Check sheet for the modelled part. Datum: model origin and axes. Units: mm. A direction names the side the tool comes from. Coordinates: 2 decimals unless noted, no trailing zeros. Write each loop counter-clockwise with the first axis right and the second up, starting at its lowest first coordinate (ties: lowest second). Pieces come first, ordered by that corner, then holes. Notation, with made-up numbers: (51, 18) - (80, 18) arc R19 ccw to (80, 24) - close; hole circle Ø4 at (-24.5, 40). An arc over 180 degrees is marked (long way). Answer as CSV lines item,"result". Start each with the question number.
from build123d import *

# Parameters (mm, degrees)
SKETCH1_W               = 25
SKETCH1_H               = 10
BOSS_EXTRUDE1_DEPTH     = 3
SKETCH2_R               = 1.25
CUT_EXTRUDE1_DEPTH      = 10
SKETCH3_W               = 10
SKETCH3_H               = 3
BOSS_EXTRUDE2_DEPTH     = 3
SKETCH4_W               = 3
SKETCH4_H               = 19.36
BOSS_EXTRUDE3_DEPTH     = 10
BOSS_EXTRUDE4_DEPTH     = 3
SKETCH6_W               = 3
SKETCH6_H               = 25
BOSS_EXTRUDE5_DEPTH     = 23
SKETCH7_W               = 3
SKETCH7_H               = 15.439035089
BOSS_EXTRUDE6_DEPTH     = 5
BOSS_EXTRUDE7_DEPTH     = 2.9
BOSS_EXTRUDE8_DEPTH     = 10
CUT_EXTRUDE2_DEPTH      = 10
CUT_EXTRUDE3_DEPTH      = 42.797000958
CUT_EXTRUDE3_DEPTH_BACK = 42.797000958
SKETCH11_R              = 1.25
SKETCH12_R              = 1.6
CUT_EXTRUDE4_DEPTH      = 40


with BuildPart() as part:
    # Sketch1 → Boss-Extrude1 (new body)
    with BuildSketch(Plane(origin=(0, 0, 0), x_dir=(1, 0, 0), z_dir=(0, 1, 0))):
        Rectangle(SKETCH1_W, SKETCH1_H)
    extrude(amount=BOSS_EXTRUDE1_DEPTH)

    # Sketch2 → Cut-Extrude1 (cut)
    with BuildSketch(Plane(origin=(0, 3, 0), x_dir=(1, 0, 0), z_dir=(0, 1, 0))):
        with Locations(Location((-4.894136616, -1.366933975, 0), (0, 0, 270))):
            Circle(SKETCH2_R)
        with Locations(Location((4.605863384, -1.366933975, 0), (0, 0, 270))):
            Circle(SKETCH2_R)
    extrude(amount=-CUT_EXTRUDE1_DEPTH, mode=Mode.SUBTRACT)

    # Sketch3 → Boss-Extrude2 (add)
    with BuildSketch(Plane.ZY.offset(12.5)):
        with Locations((0, 1.5)):
            Rectangle(SKETCH3_W, SKETCH3_H)
    extrude(amount=BOSS_EXTRUDE2_DEPTH)

    # Sketch4 → Boss-Extrude3 (add)
    with BuildSketch(Plane(origin=(0, 0, -5), x_dir=(-1, 0, 0), z_dir=(0, 0, -1))):
        with Locations((14, -9.68)):
            Rectangle(SKETCH4_W, SKETCH4_H)
    extrude(amount=-BOSS_EXTRUDE3_DEPTH)

    # Sketch5 → Boss-Extrude4 (add)
    with BuildSketch(Plane.ZY.offset(15.5)):
        Polygon((5, -19.36), (5, -22.36), (-17.439050417, -22.36), (-20.439050417, -22.36), (-20.439050417, -19.359965116), (-17.439050417, -19.359965116), align=None)
    extrude(amount=-BOSS_EXTRUDE4_DEPTH)

    # Sketch6 → Boss-Extrude5 (add)
    with BuildSketch(Plane(origin=(-12.5, 0, 0), x_dir=(0, 0, -1), z_dir=(1, 0, 0))):
        with Locations((18.939050417, -19.359753222)):
            Rectangle(SKETCH6_W, SKETCH6_H)
    extrude(amount=BOSS_EXTRUDE5_DEPTH)


with BuildPart() as boss_extrude6_tool:
    # Sketch7 → Boss-Extrude6 (new body)
    with BuildSketch(Plane(origin=(0, -19.359992227, -3.0098e-05), x_dir=(1, 0, 0), z_dir=(0, 0.9999999999987916, 1.5546330463646684e-06))):
        with Locations((-14, 12.719522209)):
            Rectangle(SKETCH7_W, SKETCH7_H)
    extrude(amount=BOSS_EXTRUDE6_DEPTH)


with BuildPart() as part_1:
    add(part.part)


with BuildPart() as part_2:
    # Boss-Extrude6: joined with boss_extrude6_tool
    add(part_1.part.fuse(boss_extrude6_tool.part, tol=0.00001))

    # Sketch8 → Boss-Extrude7 (add)
    with BuildSketch(Plane(origin=(-12.5, 0, 0), x_dir=(0, 0, -1), z_dir=(1, 0, 0))):
        Polygon((17.439050417, -22.36), (-5, -22.36), (-5, 0), (5, 0), (5.000026988, -14.359984454), (17.439050417, -14.359962784), align=None)
    extrude(amount=BOSS_EXTRUDE7_DEPTH)

    # Sketch9 → Boss-Extrude8 (add)
    with BuildSketch(Plane(origin=(0, 0, -5), x_dir=(-1, 0, 0), z_dir=(0, 0, -1))):
        Polygon((1, 1.140246778), (15.5, 1.140246778), (15.5, 4.140246778), (-12.5, 4.140246778), (-12.5, 1.140246778), align=None)
    extrude(amount=-BOSS_EXTRUDE8_DEPTH)

    # Sketch10 → Cut-Extrude2 (cut)
    with BuildSketch(Plane(origin=(0, 0, -5), x_dir=(-1, 0, 0), z_dir=(0, 0, -1))):
        Polygon((-10.464750731, 1.14), (9.6, 1.14), (9.6, 0), (-12.5, 0), (-12.5, 1.14), align=None)
    extrude(amount=-CUT_EXTRUDE2_DEPTH, mode=Mode.SUBTRACT)

    # Sketch11 → Cut-Extrude3 (cut, two sides: drawn at the far end of the back side and taken through both)
    with BuildSketch(Plane.XZ.offset(-1.14).offset(-CUT_EXTRUDE3_DEPTH_BACK)):
        with Locations(Location((-4.894136616, 1.366933975, 0), (0, 0, 90))):
            Circle(SKETCH11_R)
        with Locations(Location((4.605863384, 1.366933975, 0), (0, 0, 90))):
            Circle(SKETCH11_R)
    extrude(amount=CUT_EXTRUDE3_DEPTH + CUT_EXTRUDE3_DEPTH_BACK, mode=Mode.SUBTRACT)

    # Sketch12 → Cut-Extrude4 (cut)
    with BuildSketch(Plane.ZY.offset(15.5)):
        with Locations((-1.8211e-05, -18.359986331)):
            Circle(SKETCH12_R)
        with Locations((-10.000013494, -18.359992227)):
            Circle(SKETCH12_R)
    extrude(amount=-CUT_EXTRUDE4_DEPTH, mode=Mode.SUBTRACT)


solid = part_2.part
(1) Cross-section at B-B on y = -12. Record the boundary of the cut face in (x, z).
(2) Cross-section at A-A on x = 2. Record the boundary of the cut face in (y, z), plus the area to 3 significant figures.
(3) Go/stop test with flat-tipped pins: P1, Ø2, axis at x = -4.89, z = 1.37, coming from the -Y side; P2, Ø2.5, axis at y = -25.5, z = -19.5, coming from the +X side; P3, Ø0.9, axis at x = -14, z = -13.5, coming from the +Y side; P4, Ø2.5, axis at x = 2, z = -19.5, coming from the +Y side. Record where each tip stops, or that it passes through.
(4) Tool access check on faces 4 (the face through (1, 1.14, 0)), 5 (the face through (-12.5, -27, -19)), 6 (the face through (-9.6, -13, -4)). Record the directions out of +Z, -Z, +X, -X, +Y, -Y that give a thin tool (end or side, any length) a straight path to the whole face; none if there is none.
(5) Material ranges on probe 1 along Z at (x, y) = (-12.25, -17); probe 2 along Y at (x, z) = (-1, 0.25); probe 3 along X at (y, z) = (-7.5, -1), recorded low to high. Write a range as from..to.
(6) Release check for a two-part mould opening along Z. For faces 1 (the face through (-1, -31.86, -19)), 2 (the face through (-12.59, -19.33, -11.27)), 3 (the face through (-10, -7, 5)) record: pulls with the +Z half, pulls with the -Z half, needs draft (parallel to the pull), parting line crosses it, or undercut.
Checked values:
1,outline,"(-15.5, -5) - (-9.6, -5) - (-9.6, 5) - (-15.5, 5) - close; (-12.5, -20.44) - (10.5, -20.44) - (10.5, -17.44) - (-12.5, -17.44) - close"
2,outline,"(-31.86, -20.44) - (-6.86, -20.44) - (-6.86, -17.44) - (-31.86, -17.44) - close; (1.14, -5) - (4.14, -5) - (4.14, 5) - (1.14, 5) - close"
2,area,"105 mm^2"
3,P1,"through"
3,P2,"x = 10.5"
3,P3,"y = -14.36"
3,P4,"y = -6.86"
4,face 4,"+Z, -Z, +X, -Y"
4,face 5,"+Z, -Z, -X, -Y"
4,face 6,"+Z, +X, -Y"
5,probe 1,"-20.44..-10.84, -9.16..-0.84, 0.84..5"
5,probe 2,"1.14..4.14"
5,probe 3,"-15.5..-9.6"
6,face 1,"needs draft"
6,face 2,"undercut"
6,face 3,"pulls with the +Z half"
